```python
from build123d import *

# Parameters (mm, degrees)
SKETCH1_W                                       = 84
SKETCH1_H                                       = 20
BOSS_EXTRUDE1_DEPTH                             = 5
CSK_FOR_M3_FLAT_HEAD_MACHINE_SCREW1_D           = 3.4
CSK_FOR_M3_FLAT_HEAD_MACHINE_SCREW1_DEPTH       = 12
CSK_FOR_M3_FLAT_HEAD_MACHINE_SCREW1_CSINK_D     = 7.3
CSK_FOR_M3_FLAT_HEAD_MACHINE_SCREW1_CSINK_ANGLE = 90
CSK_FOR_M3_FLAT_HEAD_MACHINE_SCREW1_TIP         = 1.021463052


with BuildPart() as part:
    # Sketch1 → Boss-Extrude1 (new body)
    with BuildSketch(Plane.XY):
        Rectangle(SKETCH1_W, SKETCH1_H)
    extrude(amount=BOSS_EXTRUDE1_DEPTH)

    # CSK for M3 Flat Head Machine Screw1
    with Locations(Plane.XY.offset(5)):
        with Locations((38.153654124, 5.5), (38.153654124, -5.5), (-37.758420274, 5.5), (-37.758420274, -5.5)):
            CounterSinkHole(CSK_FOR_M3_FLAT_HEAD_MACHINE_SCREW1_D / 2, CSK_FOR_M3_FLAT_HEAD_MACHINE_SCREW1_CSINK_D / 2, depth=CSK_FOR_M3_FLAT_HEAD_MACHINE_SCREW1_DEPTH, counter_sink_angle=CSK_FOR_M3_FLAT_HEAD_MACHINE_SCREW1_CSINK_ANGLE)
            with Locations((0, 0, -(CSK_FOR_M3_FLAT_HEAD_MACHINE_SCREW1_DEPTH + CSK_FOR_M3_FLAT_HEAD_MACHINE_SCREW1_TIP / 2))):  # 118° drill point
                Cone(0, CSK_FOR_M3_FLAT_HEAD_MACHINE_SCREW1_D / 2, CSK_FOR_M3_FLAT_HEAD_MACHINE_SCREW1_TIP, mode=Mode.SUBTRACT)


solid = part.part
```
Could you check a few things on this model? Use its own coordinates, in mm. Round coordinates to 2 decimals unless told otherwise and drop trailing zeros. Write each loop counter-clockwise with the first axis right and the second up, starting at its lowest first coordinate (ties: lowest second). Pieces come first, ordered by that corner, then holes.
(1) Suppose I cut it at A-A on z = 2.05. Write out the boundary of the cut face in (x, y), and give its area (3 significant figures).
Findings below:
outline: (-42, -10) - (42, -10) - (42, 10) - (-42, 10) - close; hole circle Ø3.4 at (-37.76, -5.5); hole circle Ø3.4 at (-37.76, 5.5); hole circle Ø3.4 at (38.15, -5.5); hole circle Ø3.4 at (38.15, 5.5)
area: 1,640 mm2
(2) If I drill on probe 1 along X at (y, z) = (5.5, 2.45); probe 2 along X at (y, z) = (-5.75, 3.85), over which ranges is the centre line in solid material (lowest first)?
Findings below:
probe 1: x = -42 to -39.46, -36.06 to 36.45, 39.85 to 42
probe 2: x = -42 to -40.25, -35.27 to 35.67, 40.64 to 42
(3) For pin 1 (5.5 mm diameter, centred on x = -37.76, y = -5.5, fed in from +Z); pin 2 (3 mm diameter, centred on x = -37.76, y = 5.5, fed in from -Z) (3 decimals), each with a flat end and sliding along its axis, tell me the tip position at first contact or that it passes through.
Findings below:
pin 1: stops at z = 4.1
pin 2: passes through
(4) Thinking about a two-plate mould opening in Y: for faces 1 (the face through (36.583, 4.849, 1.504)), 2 (the face through (-1, 10, 2)), 3 (the face through (-42, 0, 2)), which applies, +Y half, -Y half, draft (parallel to the pull), parting line (faces both ways), or undercut?
Findings below:
face 1: undercut
face 2: +Y half
face 3: draft
(5) Suppose I cut it at B-B on y = 5.5. Write out the boundary of the cut face in (x, z).
Findings below:
outline: (-42, 0) - (-39.46, 0) - (-39.46, 3.05) - (-41.41, 5) - (-42, 5) - close; (-36.06, 0) - (36.45, 0) - (36.45, 3.05) - (34.5, 5) - (-34.11, 5) - (-36.06, 3.05) - close; (39.85, 0) - (42, 0) - (42, 5) - (41.8, 5) - (39.85, 3.05) - close
